The drawing under review shows one solid part. Ordinate dimensions are in mm from its lowest x, y, z. A direction names the side the tool comes from. Give positions to 0.01 mm unless a question says otherwise; leave off trailing zeros. Loops run counter-clockwise (first coordinate to the right, second up) from the corner with the lowest first, then second, coordinate; pieces in that order, holes last. Notation, with made-up numbers: M 89.25,24 L 132.25,24 A27 cw 132.25,62 Z; hole C 48.5,10 d10. An arc over 180 degrees is marked long. Put each result on its own line as item: value. Start each with the question number.
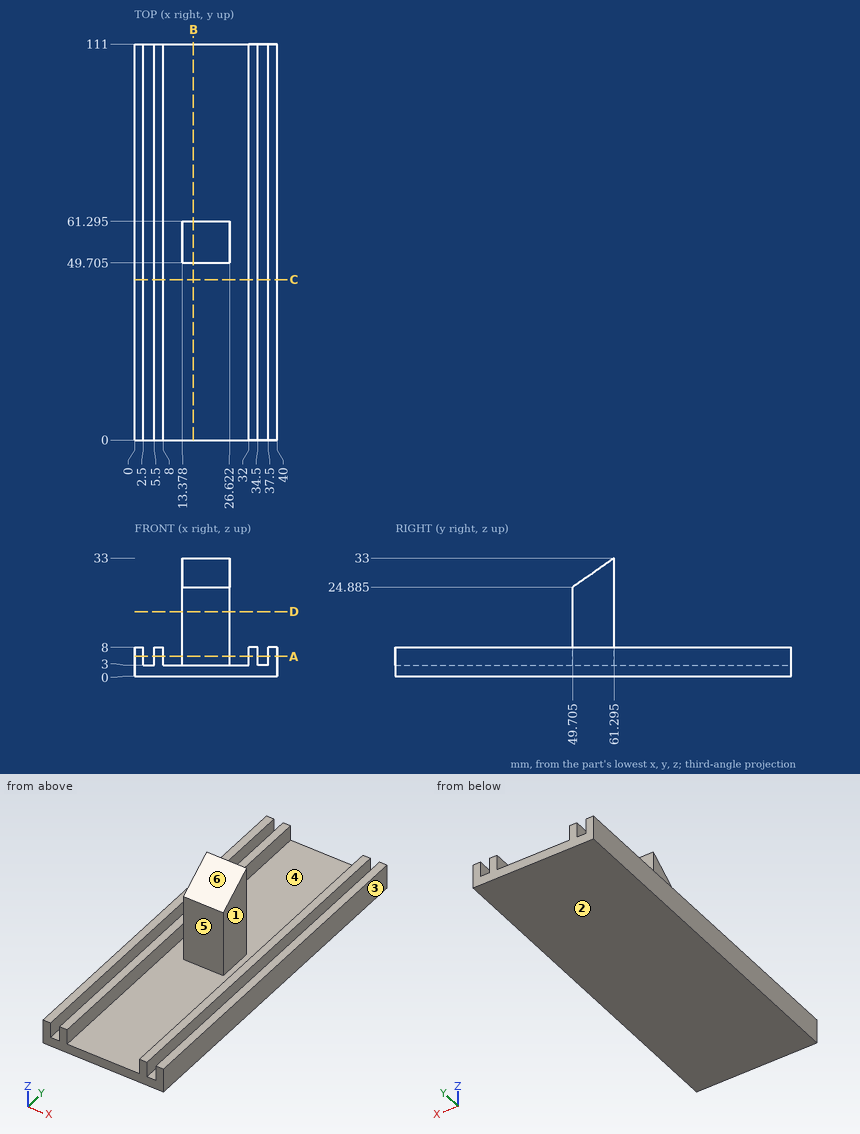
Item 1: Draft analysis for pull direction X (two halves, no side actions). For the marked faces 3, 4, 5 and 6, state which applies: +X half, -X half, draft (parallel to the pull), parting line (faces both ways), or undercut.
Item 2: Tool access review of the marked faces 1 and 2: name each direction out of +Z, -Z, +X, -X, +Y, -Y from which nothing blocks a thin tool from reaching the whole face with its end or side.
Item 3: Consider section B-B, the plane x = 16.5. Write out the cut boundary in (y, z) (1 decimal).
Item 4: Consider section A-A, the plane z = 5.5. Write out the cut boundary in (x, y) (1 decimal).
Item 5: To check wall thickness, follow L1, parallel to Z at x = 32.5, y = 58.5; L2, parallel to Z at x = 13.5, y = 84; L3, parallel to X at y = 58, z = 11. State the ranges of each line that lie inside material, in increasing order. Write a range as [from, to].
Item 6: Consider section D-D, the plane z = 18. Write out the cut boundary in (x, y) (1 decimal), plus the area to 4 significant figures.
Item 7: Consider section C-C, the plane y = 45. Write out the cut boundary in (x, z), plus the area to 3 significant figures.
Item 8: Clearance check with flat-ended pins moving along their axes: pin 1 Ø5 at (x, y) = (17.5, 13.5) entering from +Z; pin 2 Ø5 at (x, z) = (16.5, 21) entering from -Y (1 decimal); pin 3 Ø14.5 at (x, z) = (20, 23) entering from +Y (1 decimal). State where each tip first meets the part, or that it passes through.
Report:
1. face 3: +X half
1. face 4: undercut
1. face 5: undercut
1. face 6: draft
2. face 1: +Z, +Y, -Y
2. face 2: -Z, +X, -X, +Y, -Y
3. outline: M 0,0 L 111,0 L 111,3 L 61.3,3 L 61.3,33 L 49.7,24.9 L 49.7,3 L 0,3 Z
4. outline: M 0,0 L 2.5,0 L 2.5,111 L 0,111 Z; M 5.5,0 L 8,0 L 8,111 L 5.5,111 Z; M 13.4,49.7 L 26.6,49.7 L 26.6,61.3 L 13.4,61.3 Z; M 32,0 L 34.5,0 L 34.5,111 L 32,111 Z; M 37.5,0 L 40,0 L 40,111 L 37.5,111 Z
5. L1: [0, 8]
5. L2: [0, 3]
5. L3: [13.38, 26.62]
6. outline: M 13.4,49.7 L 26.6,49.7 L 26.6,61.3 L 13.4,61.3 Z
6. area: 153.5 mm²
7. outline: M 0,0 L 40,0 L 40,8 L 37.5,8 L 37.5,3 L 34.5,3 L 34.5,8 L 32,8 L 32,3 L 8,3 L 8,8 L 5.5,8 L 5.5,3 L 2.5,3 L 2.5,8 L 0,8 Z
7. area: 170 mm²
8. pin 1: z = 3
8. pin 2: y = 49.7
8. pin 3: y = 61.3
